Autodesk Inventor part; units mm, degrees
ref_plane "YZ Plane" through (0, 0, 0) normal (1, 0, 0) x (0, 1, 0)
ref_plane "XZ Plane" through (0, 0, 0) normal (0, 1, 0) x (-1, 0, 0)
ref_plane "XY Plane" through (0, 0, 0) normal (0, 0, 1) x (1, 0, 0)
sketch "スケッチ7" plane through (0, 1.5, 0) normal (0, 1, 0) x (1, 0, 0)
  line L0 (-20, 0) -> (-19.9, 0)
  line L1 (-19.9, 0) -> (-19.9, -10.2)
  line L2 (-19.9, -10.2) -> (-20, -10.2)
  line L3 (-20, -10.2) -> (-20, 0)
  line L4 (17.5, 0) -> (20, 0)
  line L5 (20, 0) -> (19.9, 0)
  line L6 (19.9, 0) -> (19.9, -10.2)
  line L7 (19.9, -10.2) -> (20, -10.2)
  line L8 (20, -10.2) -> (20, 0)
  line L9 (-20, -10.2) -> (-21.5, -10.2)
  line L10 (-20, 0) -> (-20, -1.3755)
  point P0 (0, 0)
  dimension "d21" = 0.1
  dimension "d22" = 0.1
sketch "スケッチ1" plane through (0, 0, 0) normal (0, 1, 0) x (-1, 0, 0)
  line L0 (21.5, 0) -> (-21.5, 0)
  line L1 (-21.5, 0) -> (-21.5, 25.1)
  line L2 (-21.5, 25.1) -> (21.5, 25.1)
  line L3 (21.5, 25.1) -> (21.5, 0)
  point P0 (0, 0)
  point P1 (0, 0)
  dimension "d0" = 25.1
  dimension "d1" = 43
extrude "プレート1" add sketch "スケッチ1" along normal blind 1.5
sketch "スケッチ3" plane through (0, 1.5, 0) normal (0, 1, 0) x (1, 0, 0)
  line L0 (21.5, 0) -> (-21.5, 0)
  line L1 (-20, 0) -> (-20, -17.1)
  line L2 (20, 0) -> (20, -17.1)
  line L3 (-21.5, -25.1) -> (-21.5, 0)
  line L4 (21.5, 0) -> (21.5, -25.1)
  line L5 (-20, -17.1) -> (20, -17.1)
  line L6 (-20, 0) -> (-17.5, 0)
  line L7 (-17.5, 0) -> (-17.5, -10.2)
  line L8 (-17.5, -10.2) -> (-20, -10.2)
  line L9 (-20, -10.2) -> (-20, 0)
  line L10 (20, 0) -> (17.5, 0)
  line L11 (17.5, 0) -> (17.5, -10.2)
  line L12 (17.5, -10.2) -> (20, -10.2)
  line L13 (20, -10.2) -> (20, 0)
  line L14 (-20, -10.2) -> (-21.5, -10.2)
  line L15 (20, -10.2) -> (21.5, -10.2)
  line L16 (21.5, -25.1) -> (-21.5, -25.1)
  arc A0 (-17.5, -10.2) -> (17.5, -10.2) centre (0, 8.542) ccw
  point P0 (0, 0)
  point P1 (20, -10.2)
  point P2 (17.5, 0)
  point P3 (-17.5, 0)
  dimension "d5" = 1.5
  dimension "d6" = 1.5
  dimension "d7" = 2.5
  dimension "d8" = 10.2
  dimension "d9" = 8
extrude "押し出し2" cut sketch "スケッチ3" against normal through all contours L4 L15 L2 L0 | L11 A0 L7 L0 | L1 L14 L3 L0
sketch "スケッチ4" plane through (-21.5, 0, 25.1) normal (-1, 0, 0) x (0, 0, 1)
  line L0 (-0.5569, 2.6) -> (-0.5569, 0)
  line L1 (0, 0) -> (-14.9, 0)
  line L2 (-14.9, 1.5) -> (-14.9, 0)
  line L3 (-14.9, 0) -> (0, 0)
  line L4 (0, 0) -> (0, 1.5)
  line L5 (0, 1.5) -> (-14.9, 1.5)
  point P0 (-25.1, 0)
  point P1 (0, 0)
  point P2 (-0.5569, 1.5)
extrude "押し出し3" cut sketch "スケッチ4" against normal through all contours L5 L4 L1 L0
sketch "スケッチ5" plane through (0, 1.5, 0) normal (0, 1, 0) x (1, 0, 0)
  circle A0 centre (0, -21.5431) radius 0.8
  circle A1 centre (-13, -21.5431) radius 0.8
  circle A2 centre (13, -21.5431) radius 0.8
  line L0 (-21.5, -24.5431) -> (-21.5, -10.2)
  line L1 (-21.5, -23.5431) -> (21.5, -23.5431)
  line L2 (21.5, -24.5431) -> (-21.5, -24.5431)
  line L3 (21.5, -10.2) -> (21.5, -24.5431)
  point P0 (0, 0)
  dimension "d16" = 1
extrude "切り取り1" cut sketch "スケッチ5" against normal blind 1.5
sketch "スケッチ6" plane through (0, 1.5, 0) normal (0, 1, 0) x (1, 0, 0)
  circle A0 centre (19.5, -2) radius 0.8
  circle A1 centre (19.5, -8) radius 0.8
  line L0 (0, -21.3988) -> (0, 0)
  circle A2 centre (-19.5, -2) radius 0.8
  circle A3 centre (-19.5, -8) radius 0.8
  line L1 (-20, 0) -> (-17.5, 0)
  line L2 (-20, 0) -> (-19.9, 0)
  line L3 (-19.9, 0) -> (-19.9, -10.2)
  line L4 (-19.9, -10.2) -> (-20, -10.2)
  line L5 (-20, -10.2) -> (-20, 0)
  line L6 (-20, -10.2) -> (-21.5, -10.2)
  line L7 (20, 0) -> (19.9, 0)
  line L8 (19.9, 0) -> (19.9, -10.2)
  line L9 (19.9, -10.2) -> (20, -10.2)
  line L10 (20, -10.2) -> (20, 0)
  line L11 (17.5, 0) -> (20, 0)
  line L12 (21.5, -10.2) -> (20, -10.2)
  line L13 (20, -10.2) -> (20, 0)
  dimension "d19" = 0.1
  dimension "d20" = 0.1
extrude "切り取り2" cut sketch "スケッチ6" against normal blind 1.5 contours A0 L10 | L10 A0 L8 | L8 A0 | L10 A1 L8 | A1 L10 | L8 A1 | A2 L3 | L3 A2 L5 | L5 A2 | L3 A3 L5 | A3 L3 | L5 A3
sheet face with bend "面2" sketch "スケッチ7" thickness 1.5 toward (0, -1, 0) bend radius 1.5
bend "曲げ1"
equation "\"d6\" = d5"
equation "\"d14\" = Thickness"
equation "\"d17\" = Thickness"
equation "\"d2\" = Thickness"
equation "\"d23\" = BendRadius"
equation "\"d24\" = BendReliefWidth"
equation "\"d26\" = MinimumRemnant"
equation "\"d25\" = BendReliefDepth"
equation "\"d27\" = TransitionRadius"
equation "\"BendRadius\" = Thickness"
equation "\"BendReliefWidth\" = Thickness"
equation "\"BendReliefDepth\" = 0.5 * Thickness"
equation "\"CornerReliefSize\" = 4 * Thickness"
equation "\"MinimumRemnant\" = 2 * Thickness"
equation "\"TransitionRadius\" = BendRadius"
equation "\"JacobiRadiusSize\" = BendRadius"
equation "\"GapSize\" = Thickness"
properties part number "chest_cover_base" material "アルミニウム 6061"
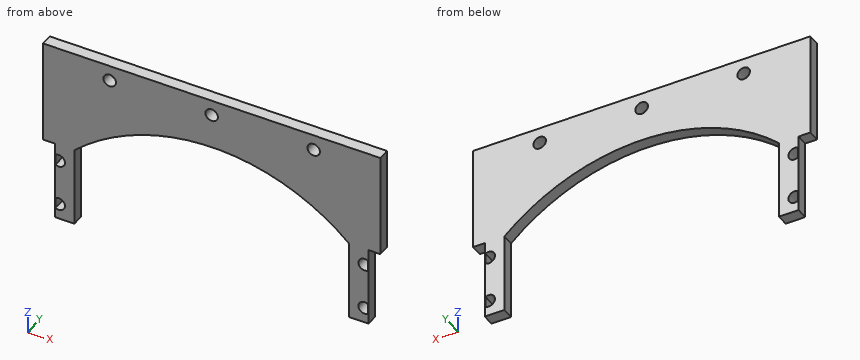
Model file for the job. Use its own axes, mm. Give positions to 0.01 mm unless a question says otherwise; leave off trailing zeros. Write each loop counter-clockwise with the first axis right and the second up, starting at its lowest first coordinate (ties: lowest second). Pieces come first, ordered by that corner, then holes. Notation, with made-up numbers: M -37,-37.5 L 22,-37.5 A12 ccw 22,-18.5 Z; hole C 60,66.25 d10. An arc over 180 degrees is marked long. One line per item, written item: value. Start each with the question number.
Q1. Saw through at B-B, the plane z = 2. Write the cut outline in (x, y), plus the area to 3 significant figures.
Q2. Drop a flat-ended pin along its axis: pin 1 Ø0.7 at (y, z) = (1, 2) entering from -X. Give the stop position or say it passes through.
Q3. Saw through at A-A, the plane x = -19.5. Write the cut outline in (y, z).
Q4. Saw through at C-C, the plane x = 0. Write the cut outline in (y, z), plus the area to 3 significant figures.
Q5. Probe probe 1 along Z at (x, y) = (-19.5, 0.75); probe 2 along X at (y, z) = (0.2, 6.5); probe 3 along Z at (x, y) = (-13, 1.15). List the from-to ranges inside material, lowest first. Write a range as [from, to].
Q6. Saw through at D-D, the plane z = 9.25. Write the cut outline in (x, y), plus the area to 3 significant figures.
Output values:
1. outline: M -20,0 L -19.9,0 L -19.9,1.5 L -20,1.5 Z; M -18.7,0 L -17.5,0 L -17.5,1.5 L -18.7,1.5 Z; M 17.5,0 L 18.7,0 L 18.7,1.5 L 17.5,1.5 Z; M 19.9,0 L 20,0 L 20,1.5 L 19.9,1.5 Z
1. area: 3.90 mm²
2. pin 1: stops at x = -20
3. outline: M 0,0 L 1.5,0 L 1.5,1.2 L 0,1.2 Z; M 0,2.8 L 1.5,2.8 L 1.5,7.2 L 0,7.2 Z; M 0,8.8 L 1.5,8.8 L 1.5,23.54 L 0,23.54 Z
4. outline: M 0,17.1 L 1.5,17.1 L 1.5,20.74 L 0,20.74 Z; M 0,22.34 L 1.5,22.34 L 1.5,23.54 L 0,23.54 Z
4. area: 7.26 mm²
5. probe 1: z = [0, 1.2], [2.8, 7.2], [8.8, 23.54]
5. probe 2: x = [-20, -17.5], [17.5, 20]
5. probe 3: z = [13.56, 20.74], [22.34, 23.54]
6. outline: M -20,0 L -17.5,0 L -17.5,1.5 L -20,1.5 Z; M 17.5,0 L 20,0 L 20,1.5 L 17.5,1.5 Z
6. area: 7.50 mm²
